Input: part model. Units: mm. Frame: model coordinates. Face numbers are marked on the shaded views. A direction names the side the tool comes from. Round coordinates to 2 decimals unless told otherwise and drop trailing zeros. Order: outer loops, then holes, each group sorted by start corner. A loop starts at its lowest first (then second) coordinate and runs counter-clockwise, first axis right, second up.
Item 1: Cut plane B-B on x = 23.5. Output: boundary loops of the cut face in (y, z), then the cut area to 3 significant figures.
Item 2: Cut plane A-A on y = 69. Output: boundary loops of the cut face in (x, z).
Item 3: First-contact query: pin 1 (10 mm diameter, centred on y = 52.5, z = -7.5, fed in from -X); pin 2 (5 mm diameter, centred on y = 40, z = -3, fed in from -X); pin 3 (4 mm diameter, centred on x = 28, y = 57.5, fed in from -Z); pin 4 (4 mm diameter, centred on x = 24.5, y = 70.5, fed in from -Z). Flat tips, straight axial feed; report the tip coordinate or a pass-through.
Item 4: Cut plane C-C on y = 53. Output: boundary loops of the cut face in (x, z), then the cut area to 3 significant figures.
Item 5: Reachability of the marked faces 1, 2 and 3 from +Z, -Z, +X, -X, +Y, -Y: full face, straight path, thin tool, end or side. Return the list, or none.
Item 6: Mould query, pull axis Z, two halves, no side actions, for the marked faces 4 and 5. Classes: released by +Z, released by -Z, zero draft, split by the parting line, or undercut.
Item 7: Cut plane D-D on x = 27. Give the number of separate pieces and of enclosed holes in the cut face, then the cut area to 3 significant figures.
Item 8: Line query: L1, parallel to Y at x = 30, z = 5.5; L2, parallel to X at y = 72, z = -5.5; L3, parallel to X at y = 40, z = -7. Output: solid intervals per line, ascending.
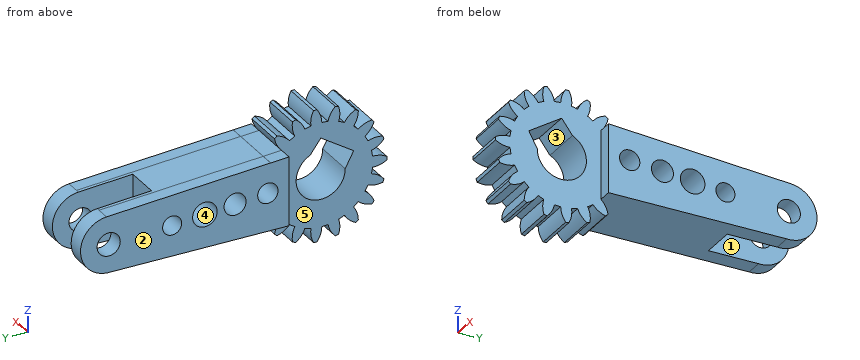
```python
from build123d import *

# Parameters (mm, degrees)
SPUR_START             = -32.726855157
SPUR_GEAR_GB_OUTLINE_R = 22.5
SPUR_GEAR_GB_DEPTH     = 75
SKETCH_2_R             = 56.152658256
CUT_EXTRUDE_1_DEPTH    = 45
EXTRUDE_1_DEPTH        = 30
EXTRUDE_START          = -30
SKETCH_5_R             = 22.5
EXTRUDE_2_DEPTH        = 30
SCALE_1_SCALE          = 0.2
CUT_EXTRUDE_3_DEPTH    = 10
EXTRUDE_3_DEPTH        = 5
SKETCH_8_R             = 1.65
CUT_EXTRUDE_4_DEPTH    = 10
SKETCH_9_W             = 18.454746183
SKETCH_9_H             = 13.449677925
CUT_EXTRUDE_5_DEPTH    = 2.5
SKETCH_10_R            = 1.446114005
SKETCH_10_R_2          = 1.567494057
SKETCH_10_R_3          = 1.749983797
SKETCH_10_R_4          = 1.35600832
CUT_EXTRUDE_6_DEPTH    = 80.014451116


# Read off the part's stored shape, not the designer's step: spur gear_gb
with BuildPart() as part:
    # spur gear_gb outline → spur gear_gb (new body)
    with BuildSketch(Plane.YZ.offset(SPUR_START)):
        with BuildLine():
            ThreePointArc((32.862431273, 33.858374177), (32.001554259, 34.671025411), (31.120587981, 35.461853886))
            ThreePointArc((31.120587981, 35.461853886), (26.170323532, 33.302671085), (22.140322459, 29.707357493))
            ThreePointArc((22.140322459, 29.707357493), (20.304903422, 30.987038971), (18.395725829, 32.153824573))
            ThreePointArc((18.395725829, 32.153824573), (20.069385125, 37.288613083), (20.058208562, 42.689267077))
            ThreePointArc((20.058208562, 42.689267077), (18.980108815, 43.178360316), (17.890094133, 43.64029024))
            ThreePointArc((17.890094133, 43.64029024), (13.909134176, 39.99074968), (11.264886092, 35.281700885))
            ThreePointArc((11.264886092, 35.281700885), (9.113403224, 35.896086104), (6.928815473, 36.379743093))
            ThreePointArc((6.928815473, 36.379743093), (6.844528189, 41.779750883), (5.080367717, 46.884153523))
            ThreePointArc((5.080367717, 46.884153523), (3.901874073, 46.996687926), (2.720930993, 47.079662024))
            ThreePointArc((2.720930993, 47.079662024), (0.14067431, 42.335248053), (-0.831275476, 37.022762562))
            ThreePointArc((-0.831275476, 37.022762562), (-3.065675621, 36.90527335), (-5.28893955, 36.653389986))
            ThreePointArc((-5.28893955, 36.653389986), (-7.12203958, 41.733442422), (-10.448009799, 45.988452479))
            ThreePointArc((-10.448009799, 45.988452479), (-11.599189267, 45.712233197), (-12.74308724, 45.407259939))
            ThreePointArc((-12.74308724, 45.407259939), (-13.643029801, 40.082103428), (-12.837355447, 34.741871474))
            ThreePointArc((-12.837355447, 34.741871474), (-14.912540945, 33.90523961), (-16.933555907, 32.945111364))
            ThreePointArc((-16.933555907, 32.945111364), (-20.316823851, 37.154705941), (-24.844183336, 40.099227051))
            ThreePointArc((-24.844183336, 40.099227051), (-25.843300471, 39.464186729), (-26.826194241, 38.804314699))
            ThreePointArc((-26.826194241, 38.804314699), (-25.948299939, 33.475478984), (-23.452308764, 28.686197563))
            ThreePointArc((-23.452308764, 28.686197563), (-25.143401065, 27.221085091), (-26.74315873, 25.656756756))
            ThreePointArc((-26.74315873, 25.656756756), (-31.309965009, 28.539718582), (-36.548104111, 29.854666195))
            ThreePointArc((-36.548104111, 29.854666195), (-37.286889069, 28.929621306), (-38.002266845, 27.986357877))
            ThreePointArc((-38.002266845, 27.986357877), (-35.44166915, 23.231304993), (-31.525840525, 19.51196706))
            ThreePointArc((-31.525840525, 19.51196706), (-32.64958354, 17.577141651), (-33.654725342, 15.578132475))
            ThreePointArc((-33.654725342, 15.578132475), (-38.910185635, 16.822047902), (-44.291470704, 16.364927041))
            ThreePointArc((-44.291470704, 16.364927041), (-44.68986467, 15.250120552), (-45.060204171, 14.125682952))
            ThreePointArc((-45.060204171, 14.125682952), (-41.094383574, 10.459696662), (-36.183058293, 8.213350193))
            ThreePointArc((-36.183058293, 8.213350193), (-36.617677028, 6.018480201), (-36.919280256, 3.801413847))
            ThreePointArc((-36.919280256, 3.801413847), (-42.293883893, 3.271485337), (-47.235169193, 1.091832139))
            ThreePointArc((-47.235169193, 1.091832139), (-47.25, -0.091929368), (-47.235169193, -1.275690876))
            ThreePointArc((-47.235169193, -1.275690876), (-42.293883893, -3.455344074), (-36.919280256, -3.985272584))
            ThreePointArc((-36.919280256, -3.985272584), (-36.617677028, -6.202338938), (-36.183058293, -8.39720893))
            ThreePointArc((-36.183058293, -8.39720893), (-41.094383574, -10.643555399), (-45.060204171, -14.309541689))
            ThreePointArc((-45.060204171, -14.309541689), (-44.68986467, -15.433979288), (-44.291470704, -16.548785777))
            ThreePointArc((-44.291470704, -16.548785777), (-38.910185635, -17.005906639), (-33.654725342, -15.761991212))
            ThreePointArc((-33.654725342, -15.761991212), (-32.64958354, -17.761000388), (-31.525840525, -19.695825796))
            ThreePointArc((-31.525840525, -19.695825796), (-35.44166915, -23.41516373), (-38.002266845, -28.170216613))
            ThreePointArc((-38.002266845, -28.170216613), (-37.286889069, -29.113480043), (-36.548104111, -30.038524932))
            ThreePointArc((-36.548104111, -30.038524932), (-31.309965009, -28.723577319), (-26.74315873, -25.840615493))
            ThreePointArc((-26.74315873, -25.840615493), (-25.143401065, -27.404943828), (-23.452308764, -28.870056299))
            ThreePointArc((-23.452308764, -28.870056299), (-25.948299939, -33.65933772), (-26.826194241, -38.988173435))
            ThreePointArc((-26.826194241, -38.988173435), (-25.843300471, -39.648045466), (-24.844183336, -40.283085788))
            ThreePointArc((-24.844183336, -40.283085788), (-20.316823851, -37.338564677), (-16.933555907, -33.128970101))
            ThreePointArc((-16.933555907, -33.128970101), (-14.912540945, -34.089098347), (-12.837355447, -34.925730211))
            ThreePointArc((-12.837355447, -34.925730211), (-13.643029801, -40.265962164), (-12.74308724, -45.591118675))
            ThreePointArc((-12.74308724, -45.591118675), (-11.599189267, -45.896091934), (-10.448009799, -46.172311216))
            ThreePointArc((-10.448009799, -46.172311216), (-7.12203958, -41.917301159), (-5.28893955, -36.837248723))
            ThreePointArc((-5.28893955, -36.837248723), (-3.065675621, -37.089132087), (-0.831275476, -37.206621299))
            ThreePointArc((-0.831275476, -37.206621299), (0.14067431, -42.51910679), (2.720930993, -47.263520761))
            ThreePointArc((2.720930993, -47.263520761), (3.901874073, -47.180546663), (5.080367717, -47.06801226))
            ThreePointArc((5.080367717, -47.06801226), (6.844528189, -41.96360962), (6.928815473, -36.56360183))
            ThreePointArc((6.928815473, -36.56360183), (9.113403224, -36.079944841), (11.264886092, -35.465559622))
            ThreePointArc((11.264886092, -35.465559622), (13.909134176, -40.174608417), (17.890094133, -43.824148977))
            ThreePointArc((17.890094133, -43.824148977), (18.980108815, -43.362219053), (20.058208562, -42.873125814))
            ThreePointArc((20.058208562, -42.873125814), (20.069385125, -37.47247182), (18.395725829, -32.33768331))
            ThreePointArc((18.395725829, -32.33768331), (20.304903422, -31.170897707), (22.140322459, -29.891216229))
            ThreePointArc((22.140322459, -29.891216229), (26.170323532, -33.486529822), (31.120587981, -35.645712623))
            ThreePointArc((31.120587981, -35.645712623), (32.001554259, -34.854884148), (32.862431273, -34.042232914))
            ThreePointArc((32.862431273, -34.042232914), (31.119412774, -28.930572226), (27.869173851, -24.617437006))
            ThreePointArc((27.869173851, -24.617437006), (29.296052271, -22.893962115), (30.616511345, -21.087657722))
            ThreePointArc((30.616511345, -21.087657722), (35.595552259, -23.179628097), (40.978683235, -23.614472179))
            ThreePointArc((40.978683235, -23.614472179), (41.555134745, -22.58044369), (42.105499643, -21.532297832))
            ThreePointArc((42.105499643, -21.532297832), (38.797169181, -17.2635582), (34.322564452, -14.239471396))
            ThreePointArc((34.322564452, -14.239471396), (35.112519281, -12.146072463), (35.774926162, -10.008886264))
            ThreePointArc((35.774926162, -10.008886264), (41.163450577, -10.370815972), (46.396102311, -9.034199232))
            ThreePointArc((46.396102311, -9.034199232), (46.605571586, -7.869023759), (46.785783792, -6.698966145))
            ThreePointArc((46.785783792, -6.698966145), (42.270650308, -3.735731746), (37.056572625, -2.328400087))
            ThreePointArc((37.056572625, -2.328400087), (37.124, -0.091929368), (37.056572625, 2.14454135))
            ThreePointArc((37.056572625, 2.14454135), (42.270650308, 3.551873009), (46.785783792, 6.515107408))
            ThreePointArc((46.785783792, 6.515107408), (46.605571586, 7.685165023), (46.396102311, 8.850340496))
            ThreePointArc((46.396102311, 8.850340496), (41.163450577, 10.186957235), (35.774926162, 9.825027527))
            ThreePointArc((35.774926162, 9.825027527), (35.112519281, 11.962213726), (34.322564452, 14.05561266))
            ThreePointArc((34.322564452, 14.05561266), (38.797169181, 17.079699464), (42.105499643, 21.348439095))
            ThreePointArc((42.105499643, 21.348439095), (41.555134745, 22.396584953), (40.978683235, 23.430613443))
            ThreePointArc((40.978683235, 23.430613443), (35.595552259, 22.99576936), (30.616511345, 20.903798985))
            ThreePointArc((30.616511345, 20.903798985), (29.296052271, 22.710103378), (27.869173851, 24.433578269))
            ThreePointArc((27.869173851, 24.433578269), (31.119412774, 28.746713489), (32.862431273, 33.858374177))
        make_face()
        with Locations((0, -0.091929368)):
            Circle(SPUR_GEAR_GB_OUTLINE_R, mode=Mode.SUBTRACT)
    extrude(amount=SPUR_GEAR_GB_DEPTH)

    # 草图2 → 切除-拉伸1 (cut)
    with BuildSketch(Plane.ZY.offset(32.726855157)):
        with Locations((-0.091929368, 0)):
            Circle(SKETCH_2_R)
    extrude(amount=-CUT_EXTRUDE_1_DEPTH, mode=Mode.SUBTRACT)

    # 草图4 → 凸台-拉伸1 (add)
    with BuildSketch(Plane(origin=(42.273144843, 0, 0), x_dir=(0, 0, -1), z_dir=(1, 0, 0))):
        with BuildLine():
            Line((-24.433578269, 27.869173851), (-23.430613443, 40.978683235))
            Line((-23.430613443, 40.978683235), (-14.487711984, 157.869173851))
            ThreePointArc((-14.487711984, 157.869173851), (7.042421291, 176.339040577), (25.512288016, 154.808907302))
            Line((25.512288016, 154.808907302), (24.617437006, 27.869173851))
            Line((24.617437006, 27.869173851), (-24.433578269, 27.869173851))
        make_face()
    extrude(amount=-EXTRUDE_1_DEPTH)

    # 草图5 → 凸台-拉伸2 (add)
    with BuildSketch(Plane(origin=(42.273144843, 0, 0), x_dir=(0, 0, -1), z_dir=(1, 0, 0)).offset(EXTRUDE_START)):
        with Locations((0.091929368, 0)):
            Circle(SKETCH_5_R)
    extrude(amount=EXTRUDE_2_DEPTH)


with BuildPart() as part_1:
    # 缩放比例1: scaled about (27.273144843, 52.936955481, -1.705643422)
    add(part.part.scale(SCALE_1_SCALE).moved(Location((21.818515874, 42.349564385, -1.364514738))))

    # 草图6 → 切除-拉伸3 (cut)
    with BuildSketch(Plane(origin=(30.273144843, 0, 0), x_dir=(0, 0, -1), z_dir=(1, 0, 0))):
        with BuildLine():
            Line((-0.872032296, 37.645512175), (-3.855195053, 42.325601914))
            Line((-3.855195053, 42.325601914), (-1.776224322, 43.856192956))
            ThreePointArc((-1.776224322, 43.856192956), (4.342900611, 44.217290275), (1.382900611, 38.849564385))
            Line((1.382900611, 38.849564385), (-0.872032296, 37.645512175))
        make_face()
    extrude(amount=-CUT_EXTRUDE_3_DEPTH, mode=Mode.SUBTRACT)

    # 草图7 → 凸台-拉伸3 (add, symmetric)
    with BuildSketch(Plane(origin=(27.273144843, 0, 0), x_dir=(0, 0, -1), z_dir=(1, 0, 0))):
        with BuildLine():
            Line((6.288002139, 47.923399155), (6.466972341, 73.311345845))
            ThreePointArc((6.466972341, 73.311345845), (2.772998996, 77.6173725), (-1.533027659, 73.923399155))
            Line((-1.533027659, 73.923399155), (-3.321607951, 50.545301032))
            Line((-3.321607951, 50.545301032), (-3.322451181, 50.53427937))
            Line((-3.322451181, 50.53427937), (-3.522200916, 47.923399155))
            Line((-3.522200916, 47.923399155), (6.288002139, 47.923399155))
        make_face()
    extrude(amount=EXTRUDE_3_DEPTH, both=True)

    # 草图8 → 切除-拉伸4 (cut)
    with BuildSketch(Plane(origin=(32.273144843, 0, 0), x_dir=(0, 0, -1), z_dir=(1, 0, 0))):
        with Locations((2.466972341, 73.6173725)):
            Circle(SKETCH_8_R)
    extrude(amount=-CUT_EXTRUDE_4_DEPTH, mode=Mode.SUBTRACT)

    # 草图9 → 切除-拉伸5 (cut, symmetric)
    with BuildSketch(Plane(origin=(27.273144843, 0, 0), x_dir=(0, 0, -1), z_dir=(1, 0, 0))):
        with Locations((1.880211444, 72.900415106)):
            Rectangle(SKETCH_9_W, SKETCH_9_H)
    extrude(amount=CUT_EXTRUDE_5_DEPTH, both=True, mode=Mode.SUBTRACT)

    # 草图10 → 切除-拉伸6 (cut, through all)
    with BuildSketch(Plane(origin=(32.273144843, 0, 0), x_dir=(0, 0, -1), z_dir=(1, 0, 0))):
        with Locations((0.89588905, 50.944816989)):
            Circle(SKETCH_10_R)
        with Locations((1.285013172, 55.613074907)):
            Circle(SKETCH_10_R_2)
        with Locations((1.667330314, 59.914483987)):
            Circle(SKETCH_10_R_3)
        with Locations((2.056454436, 64.582741905)):
            Circle(SKETCH_10_R_4)
    extrude(amount=-CUT_EXTRUDE_6_DEPTH, mode=Mode.SUBTRACT)


solid = part_1.part
```
From the geometry:
1. outline: (47.92, -6.29) - (73.31, -6.47) arc R4.01 ccw to (73.92, 1.53) - (47.92, 3.52) - close; hole circle Ø2.89 at (50.94, -0.9); hole circle Ø3.13 at (55.61, -1.29); hole circle Ø3.5 at (59.91, -1.67); hole circle Ø2.71 at (64.58, -2.06); hole circle Ø3.3 at (73.62, -2.47)
1. area: 216 mm2
2. outline: (22.27, -6.44) - (24.77, -6.44) - (24.77, 1.91) - (22.27, 1.91) - close; (29.77, -6.44) - (32.27, -6.44) - (32.27, 1.91) - (29.77, 1.91) - close
3. pin 1: stops at x = 22.27
3. pin 2: stops at x = 24.27
3. pin 3: stops at z = -6.37
3. pin 4: stops at z = -6.46
4. outline: (22.27, -6.32) - (32.27, -6.32) - (32.27, 3.13) - (22.27, 3.13) - close
4. area: 94.6 mm2
5. face 1: +Z, -Z, +Y
5. face 2: +Z, -Z, -X, +Y, -Y
5. face 3: +X, -X
6. face 4: undercut
6. face 5: zero draft
7. separate pieces: 1
7. enclosed holes: 5
7. area: 290 mm2
8. L1: y = 37.11 to 38.79, 39.57 to 46.21, 47.95 to 48.82
8. L2: x = 22.27 to 24.77, 29.77 to 32.27
8. L3: x = 24.27 to 30.27
